```python
from build123d import *

# Parameters (mm, degrees)
SKETCH1_W           = 10
SKETCH1_H           = 50
BOSS_EXTRUDE1_DEPTH = 5.3
CUT_EXTRUDE1_DEPTH  = 3.2
SKETCH3_R           = 2
CUT_EXTRUDE2_DEPTH  = 8
SKETCH4_W           = 10
SKETCH4_H           = 5.3
BOSS_EXTRUDE2_DEPTH = 12
SKETCH5_W           = 10
SKETCH5_H           = 5.3
BOSS_EXTRUDE3_DEPTH = 12
CUT_EXTRUDE3_DEPTH  = 12
SKETCH8_W           = 6
SKETCH8_H           = 13
CUT_EXTRUDE4_DEPTH  = 3.3
SKETCH9_R           = 1.75
CUT_EXTRUDE5_DEPTH  = 3.3


with BuildPart() as part:
    # Sketch1 → Boss-Extrude1 (new body)
    with BuildSketch(Plane.XY):
        with Locations((5, 25)):
            Rectangle(SKETCH1_W, SKETCH1_H)
    extrude(amount=BOSS_EXTRUDE1_DEPTH)

    # Sketch2 → Cut-Extrude1 (cut)
    with BuildSketch(Plane.XY.offset(5.3)):
        Polygon((8.5, 14.520725942), (5, 16.541451884), (1.5, 14.520725942), (1.5, 10.479274058), (5, 8.458548116), (8.5, 10.479274058), align=None)
        Polygon((8.5, 39.520725942), (5, 41.541451884), (1.5, 39.520725942), (1.5, 35.479274058), (5, 33.458548116), (8.5, 35.479274058), align=None)
    extrude(amount=-CUT_EXTRUDE1_DEPTH, mode=Mode.SUBTRACT)

    # Sketch3 → Cut-Extrude2 (cut)
    with BuildSketch(Plane.XY.offset(2.1)):
        with Locations((5, 37.5)):
            Circle(SKETCH3_R)
        with Locations((5, 12.5)):
            Circle(SKETCH3_R)
    extrude(amount=-CUT_EXTRUDE2_DEPTH, mode=Mode.SUBTRACT)

    # Sketch4 → Boss-Extrude2 (add)
    with BuildSketch(Plane(origin=(0, 50, 0), x_dir=(1, 0, 0), z_dir=(0, 1, 0))):
        with Locations((5, -2.65)):
            Rectangle(SKETCH4_W, SKETCH4_H)
    extrude(amount=BOSS_EXTRUDE2_DEPTH)

    # Sketch5 → Boss-Extrude3 (add)
    with BuildSketch(Plane.XZ):
        with Locations((5, 2.65)):
            Rectangle(SKETCH5_W, SKETCH5_H)
    extrude(amount=BOSS_EXTRUDE3_DEPTH)

    # Sketch6 → Cut-Extrude3 (cut)
    with BuildSketch(Plane.ZY):
        Polygon((3.3, 62), (0, 47), (0, 62), align=None)
        Polygon((0, -12), (3.3, -12), (0, 3), align=None)
    extrude(amount=-CUT_EXTRUDE3_DEPTH, mode=Mode.SUBTRACT)

    # Sketch8 → Cut-Extrude4 (cut)
    with BuildSketch(Plane(origin=(0, 0, 0), x_dir=(-1, 0, 0), z_dir=(0, 0, -1))):
        with Locations((-5, 55.5)):
            Rectangle(SKETCH8_W, SKETCH8_H)
        with Locations((-5, -5.5)):
            Rectangle(SKETCH8_W, SKETCH8_H)
    extrude(amount=-CUT_EXTRUDE4_DEPTH, mode=Mode.SUBTRACT)

    # Sketch9 → Cut-Extrude5 (cut)
    with BuildSketch(Plane(origin=(0, 0, 3.3), x_dir=(-1, 0, 0), z_dir=(0, 0, -1))):
        with Locations((-5, -5)):
            Circle(SKETCH9_R)
        with Locations((-5, 55)):
            Circle(SKETCH9_R)
    extrude(amount=-CUT_EXTRUDE5_DEPTH, mode=Mode.SUBTRACT)


solid = part.part
```
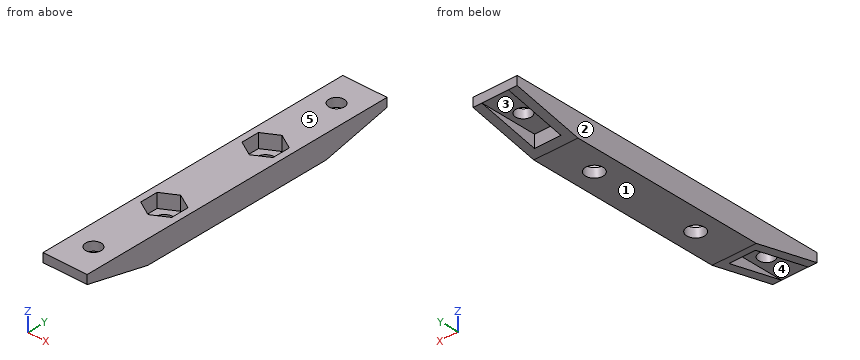
For this review, take the finished solid that the model builds, in its own axes (mm). Face numbers are marked on the shaded views. A direction names the side the tool comes from. Give positions to 0.01 mm unless a question says otherwise; leave off trailing zeros. Write each loop counter-clockwise with the first axis right and the second up, starting at its lowest first coordinate (ties: lowest second). Pieces come first, ordered by that corner, then holes.
Item 1: Machinability: for the marked faces 4 and 5, which of the approach directions +Z, -Z, +X, -X, +Y, -Y give a long, thin tool a straight path to every point of the face, cutting with its end or side? Answer none if there is none.
Item 2: Wall thickness on probe 1 along Y at (x, z) = (5, 3.8); probe 2 along Y at (x, z) = (5, 0.7); probe 3 along X at (y, z) = (35.5, 2.5): over which ranges is each line inside the solid? List them lowest first.
Item 3: The part is to be moulded in two halves that separate along X. For the marked faces 1, 2 and 3, say which applies: +X half, -X half, draft (parallel to the pull), parting line (faces both ways), or undercut.
Item 4: Take a section at A-A (y = -5). Give the boundary of the cut face in (x, z).
Item 5: Take a section at C-C (z = 1.15). Give the boundary of the cut face in (x, y).
Item 6: Insertion check: P1, Ø3.5, axis at x = 5.5, y = 38.5, coming from the +Z side; P2, Ø5, axis at x = 4, y = 56, coming from the -Z side; P3, Ø5.5, axis at x = 5, y = -5, coming from the -Z side. Each pin has a flat end and moves straight along its axis. Give the tip position at first contact, or say it passes through.
Item 7: Take a section at D-D (y = 37.5). Give the boundary of the cut face in (x, z).
Item 8: Take a section at B-B (z = 4.6). Give the boundary of the cut face in (x, y).
Established:
1. face 4: -Z, -Y
1. face 5: +Z, +X, -X, +Y, -Y
2. probe 1: y = -12 to -6.75, -3.25 to 8.46, 16.54 to 33.46, 41.54 to 53.25, 56.75 to 62
2. probe 2: y = 1 to 10.5, 14.5 to 35.5, 39.5 to 49
2. probe 3: x = 0 to 1.5, 8.5 to 10
3. face 1: draft
3. face 2: -X half
3. face 3: undercut
4. outline: (0, 1.76) - (2, 1.76) - (2, 3.3) - (3.25, 3.3) - (3.25, 5.3) - (0, 5.3) - close; (6.75, 3.3) - (8, 3.3) - (8, 1.76) - (10, 1.76) - (10, 5.3) - (6.75, 5.3) - close
5. outline: (0, -2.23) - (2, -2.23) - (2, 1) - (8, 1) - (8, -2.23) - (10, -2.23) - (10, 52.23) - (8, 52.23) - (8, 49) - (2, 49) - (2, 52.23) - (0, 52.23) - close; hole circle Ø4 at (5, 12.5); hole circle Ø4 at (5, 37.5)
6. P1: stops at z = 2.1
6. P2: stops at z = 1.65
6. P3: stops at z = 3.3
7. outline: (0, 0) - (3, 0) - (3, 2.1) - (1.5, 2.1) - (1.5, 5.3) - (0, 5.3) - close; (7, 0) - (10, 0) - (10, 5.3) - (8.5, 5.3) - (8.5, 2.1) - (7, 2.1) - close
8. outline: (0, -12) - (10, -12) - (10, 62) - (0, 62) - close; hole (1.5, 10.48) - (5, 8.46) - (8.5, 10.48) - (8.5, 14.52) - (5, 16.54) - (1.5, 14.52) - close; hole (1.5, 35.48) - (5, 33.46) - (8.5, 35.48) - (8.5, 39.52) - (5, 41.54) - (1.5, 39.52) - close; hole circle Ø3.5 at (5, -5); hole circle Ø3.5 at (5, 55)
